```python
from build123d import *

# Parameters (mm, degrees)
SKETCH_1_R               = 2.5
EXTRUDE_1_DEPTH          = 2
SKETCH_4_R               = 2.5
EXTRUDE_3_DEPTH          = 0.5
CUT_EXTRUDE_1_DEPTH      = 56.022289153
CUT_EXTRUDE_1_DEPTH_BACK = 56.022289153
SKETCH_2_R               = 2
SKETCH_3_R               = 2
EXTRUDE_2_DEPTH          = 29.25


with BuildPart() as part:
    # 草圖1 → 填料-伸長1 (new body)
    with BuildSketch(Plane.XY):
        with BuildLine():
            Line((-53.002575001, -1.246781249), (-26.890819753, -5))
            Line((-26.890819753, -5), (51.758125458, -5))
            ThreePointArc((51.758125458, -5), (54.462035166, -3.299566191), (54.100731886, -0.125914857))
            Line((54.100731886, -0.125914857), (51.200975848, 3.49878019))
            ThreePointArc((51.200975848, 3.49878019), (49.810255532, 4.605212945), (48.07750061, 5))
            Line((48.07750061, 5), (-51.758125458, 5))
            ThreePointArc((-51.758125458, 5), (-54.462035166, 3.299566191), (-54.100731886, 0.125914857))
            Line((-54.100731886, 0.125914857), (-53.002575001, -1.246781249))
        make_face()
        Circle(SKETCH_1_R, mode=Mode.SUBTRACT)
    extrude(amount=EXTRUDE_1_DEPTH)

    # 草圖4 → 填料-伸長3 (add)
    with BuildSketch(Plane.XY.offset(2)):
        with Locations((51.758125458, -2)):
            Circle(SKETCH_4_R)
    extrude(amount=EXTRUDE_3_DEPTH)

    # 草圖2 → 除料-伸長1 (cut, two sides: drawn at the far end of the back side and taken through both)
    with BuildSketch(Plane.XY.offset(2).offset(-CUT_EXTRUDE_1_DEPTH_BACK)):
        with Locations((-51.758125458, 2)):
            Circle(SKETCH_2_R)
        with Locations((51.758125458, -2)):
            Circle(SKETCH_2_R)
    extrude(amount=CUT_EXTRUDE_1_DEPTH + CUT_EXTRUDE_1_DEPTH_BACK, mode=Mode.SUBTRACT)

    # 草圖3 → 填料-伸長2 (add)
    with BuildSketch(Plane(origin=(0, 0, 2), x_dir=(-1, 0, 0), z_dir=(0, 0, -1))):
        with Locations(Location((30, 2, 0), (0, 0, 180))):
            Circle(SKETCH_3_R)
        with Locations(Location((-30, 2, 0), (0, 0, 180))):
            Circle(SKETCH_3_R)
    extrude(amount=EXTRUDE_2_DEPTH)

    # 鏡射1: part across plane


with BuildPart() as part_1:
    add(part.part)
    add(part.part.mirror(Plane(origin=(-30, 2, -27.25), x_dir=(1, 0, 0), z_dir=(0, 0, -1))))


solid = part_1.part
```
Geometry check sheet. Reference: the model listing, model coordinates, mm. A direction names the side the tool comes from. Coordinates: 2 decimals unless noted, no trailing zeros. Order: outer loops, then holes, each group sorted by start corner. A loop starts at its lowest first (then second) coordinate and runs counter-clockwise, first axis right, second up. Notation, with made-up numbers: M 74.25,47.25 L 84.25,47.25 A22 cw 84.25,69.25 Z; hole C 86,-4.75 d6. An arc over 180 degrees is marked long. One line per question, with ' | ' between items. Start each with the question number.
Item 1: Draft check along Z on faces 3 (the cylindrical face through (-28.092, 1.399, -27.632)), 4 (the flat face through (-1, 3, -56.5)), 5 (the flat face through (12, -5, 1)). Enter one of: pulls with the +Z half, pulls with the -Z half, needs draft (parallel to the pull), parting line crosses it, or undercut.
Item 2: Cross-section at B-B on z = -47.5. Enter the section's corners in (x, y), then the cut area to 3 significant figures.
Item 3: Material ranges on L1, parallel to Z at x = -30, y = -4.25; L2, parallel to Y at x = 0, z = 1; L3, parallel to Z at x = -31, y = 1.25, recorded low to high. Write a range as [from, to].
Item 4: Set-up check for faces 1 (the cylindrical face through (54.067, -2.958, -56.746)), 2 (the cylindrical face through (49.76, -1.91, 1.23)): record each of +Z, -Z, +X, -X, +Y, -Y from which the full face is reachable in a straight line by a thin tool's end or side.
Item 5: Gauge pin test, flat ends, axial feed: pin 1 (3 mm diameter, centred on x = 0, y = 0, fed in from +Z); pin 2 (3 mm diameter, centred on x = -34.5, y = 0, fed in from -Z); pin 3 (6 mm diameter, centred on x = 29, y = 2.5, fed in from +Z); pin 4 (6 mm diameter, centred on y = 0, z = -7, fed in from +X). Record the tip position at first contact, or that the pin passes through.
Item 6: Cross-section at C-C on x = 30. Enter the section's corners in (y, z), then the cut area to 3 significant figures.
Item 7: Cross-section at D-D on x = -30. Enter the section's corners in (y, z).
Item 8: Cross-section at A-A on x = 46.5. Enter the section's corners in (y, z), then the cut area to 3 significant figures.
Findings:
1) face 3: undercut | face 4: pulls with the -Z half | face 5: needs draft
2) outline: C -30,2 d4; C 30,2 d4 | area: 25.1 mm²
3) L1: z = [-56.5, -54.5], [0, 2] | L2: y = [-5, -2.5], [2.5, 5] | L3: z = [-56.5, 2]
4) face 1: -Z | face 2: +Z, -Z
5) pin 1: passes through | pin 2: stops at z = -56.5 | pin 3: stops at z = 2 | pin 4: stops at x = 32
6) outline: M -5,-56.5 L 5,-56.5 L 5,-54.5 L 4,-54.5 L 4,0 L 5,0 L 5,2 L -5,2 L -5,0 L 0,0 L 0,-54.5 L -5,-54.5 Z | area: 258 mm²
7) outline: M -4.55,-56.5 L 5,-56.5 L 5,-54.5 L 4,-54.5 L 4,0 L 5,0 L 5,2 L -4.55,2 L -4.55,0 L 0,0 L 0,-54.5 L -4.55,-54.5 Z
8) outline: M -5,-56.5 L 5,-56.5 L 5,-54.5 L -5,-54.5 Z; M -5,0 L 5,0 L 5,2 L -5,2 Z | area: 40.0 mm²
